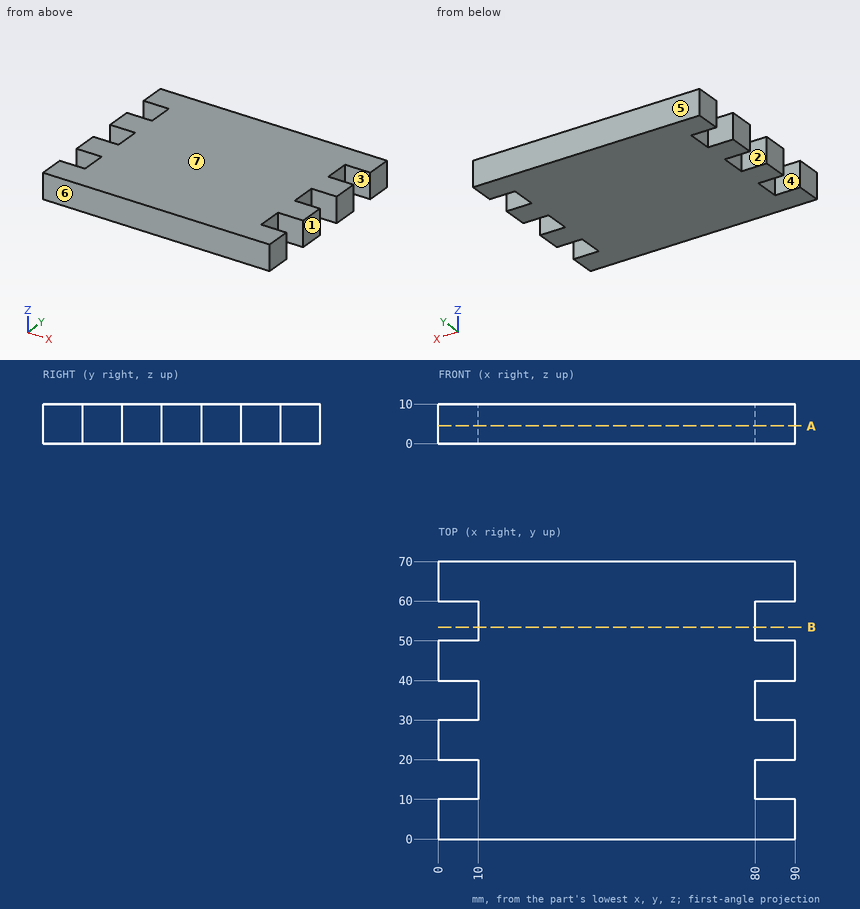
The figure shows three views and two pictorial views of one solid part (mm, origin at its lowest corner). Answer the questions. A direction names the side the tool comes from. Give positions to 0.01 mm unless a question says otherwise; leave off trailing zeros. Order: outer loops, then holes, each group sorted by start corner. A loop starts at its lowest first (then second) coordinate and runs counter-clockwise, first axis right, second up. Notation, with made-up numbers: (55.25, -11) -> (106.25, -11) arc R12 ccw to (106.25, 8) -> close; hole circle Ø10 at (58, 67.25). An arc over 180 degrees is marked (long way). Answer as a JSON object with one key per item and string values. Group by question number.
Item 1: A flat-ended cylindrical pin translates along its axis: pin 1 (3 mm diameter, centred on y = 34, z = 5.5, fed in from -X). Find the tip coordinate at first contact, or state that the pin passes through.
Item 2: Determine the mould class of the marked faces 4, 5, 6 and 7 for opening direction Y: pulls with the +Y half, pulls with the -Y half, needs draft (parallel to the pull), parting line crosses it, or undercut.
Item 3: The part is cut by section A-A on z = 4.5. Write down the section's boundary in (x, y).
Item 4: The part is cut by section B-B on y = 53.5. Write down the section's boundary in (x, z).
Item 5: A tool of negligible diameter and unlimited length cuts with its end or side. For the marked faces 1, 2 and 3, from which of +Z, -Z, +X, -X, +Y, -Y can it reach the whole face along a straight path? Write none if from no direction.
Item 6: Consider L1, parallel to X at y = 51, z = 7.25. Determine where the line is inside the solid, lowest interval first. Write a range as from..to.
Result set:
{
 "1": {"pin 1": "x = 10"},
 "2": {"face 4": "undercut", "face 5": "pulls with the +Y half", "face 6": "pulls with the -Y half", "face 7": "needs draft"},
 "3": {"outline": "(0, 0) -> (90, 0) -> (90, 10) -> (80, 10) -> (80, 20) -> (90, 20) -> (90, 30) -> (80, 30) -> (80, 40) -> (90, 40) -> (90, 50) -> (80, 50) -> (80, 60) -> (90, 60) -> (90, 70) -> (0, 70) -> (0, 60) -> (10, 60) -> (10, 50) -> (0, 50) -> (0, 40) -> (10, 40) -> (10, 30) -> (0, 30) -> (0, 20) -> (10, 20) -> (10, 10) -> (0, 10) -> close"},
 "4": {"outline": "(10, 0) -> (80, 0) -> (80, 10) -> (10, 10) -> close"},
 "5": {"face 1": "+Z, -Z, +X, +Y, -Y", "face 2": "+Z, -Z, -X", "face 3": "+Z, -Z, +X"},
 "6": {"L1": "10..80"}
}
